Part model, mm, in its own coordinate system. A direction names the side the tool comes from. Coordinates: 2 decimals unless noted, no trailing zeros. Loops run counter-clockwise (first coordinate to the right, second up) from the corner with the lowest first, then second, coordinate; pieces in that order, holes last. Notation, with made-up numbers: (60.5, 39.25) - (77.5, 39.25) arc R30 cw to (77.5, 71.25) - close; hole circle Ø5 at (-35, -23). An arc over 180 degrees is marked (long way). Use a Markdown table: item, result. Add a question column.
1) Pull direction X, two halves, no side cores. Call faces 6 (the face through (-33.8, 24.45, -11.25)), 7 (the face through (-1, 25.25, 0)), 8 (the face through (-76.25, -5, -17)), 9 (the face through (76.25, -5, -17)): +X half, -X half, draft (parallel to the pull), parting line (faces both ways), or undercut.
2) Band-saw the part on C-C (z = -16.5). Give the cut face in (x, y), plus the area to 3 significant figures.
3) Band-saw the part on A-A (y = 1.5). Give the cut face in (x, z), plus the area to 3 significant figures.
4) Drop flat-ended pins along their axis: P1, Ø6.5, axis at x = 9, z = 0, coming from the -Y side; P2, Ø10, axis at y = 8, z = -31.5, coming from the -X side. Give the stop position or say it passes through.
5) Probe probe 1 along X at (y, z) = (-13.5, -41); probe 2 along Z at (x, y) = (-67, 1); probe 3 along Y at (x, z) = (41, 4). List the from-to ranges inside material, lowest first. Write a range as [from, to].
6) Tool access for faces 1 (the face through (-75.8, 0.8, -35.7)), 2 (the face through (75.25, 0, 0)), 3 (the face through (55, 18.07, 10.76)), 4 (the face through (-75.25, -10, -25)), 5 (the face through (-1, -21, 11.25)): list every direction of +Z, -Z, +X, -X, +Y, -Y with a clear straight run to the whole face (end or side of a thin tool).
7) Band-saw the part on D-D (y = 22.5). Give the cut face in (x, z).
8) Band-saw the part on B-B (x = 5). Give the cut face in (y, z).
from build123d import *

# Parameters (mm, degrees)
SKETCH1_W           = 150.5
SKETCH1_H           = 48.5
BOSS_EXTRUDE1_DEPTH = 10.25
SHELL1_T            = 1
SKETCH2_W           = 145.5
SKETCH2_H           = 48.5
CUT_EXTRUDE1_DEPTH  = 1
CUT_EXTRUDE2_DEPTH  = 1
BOSS_EXTRUDE2_DEPTH = 1


with BuildPart() as part:
    # Sketch1 → Boss-Extrude1 (new, symmetric)
    with BuildSketch(Plane.XY):
        Rectangle(SKETCH1_W, SKETCH1_H)
    extrude(amount=BOSS_EXTRUDE1_DEPTH, both=True)

    # Shell1
    shell1_openings = [part.faces().sort_by_distance(p)[0] for p in [
        (0, -24.25, 0),
    ]]
    offset(amount=SHELL1_T, openings=shell1_openings, kind=Kind.INTERSECTION)

    # Sketch2 → Cut-Extrude1 (cut)
    with BuildSketch(Plane(origin=(0, 0, -11.25), x_dir=(-1, 0, 0), z_dir=(0, 0, -1))):
        Rectangle(SKETCH2_W, SKETCH2_H)
    extrude(amount=-CUT_EXTRUDE1_DEPTH, mode=Mode.SUBTRACT)

    # Sketch3 → Cut-Extrude2 (cut)
    with BuildSketch(Plane.XY.offset(11.25)):
        with BuildLine():
            Line((51.5, -19.5), (-51.5, -19.5))
            ThreePointArc((-51.5, -19.5), (-55.035533906, -18.035533906), (-56.5, -14.5))
            Line((-56.5, -14.5), (-56.5, 14.5))
            ThreePointArc((-56.5, 14.5), (-55.035533906, 18.035533906), (-51.5, 19.5))
            Line((-51.5, 19.5), (51.5, 19.5))
            ThreePointArc((51.5, 19.5), (55.035533906, 18.035533906), (56.5, 14.5))
            Line((56.5, 14.5), (56.5, -14.5))
            ThreePointArc((56.5, -14.5), (55.035533906, -18.035533906), (51.5, -19.5))
        make_face()
    extrude(amount=-CUT_EXTRUDE2_DEPTH, mode=Mode.SUBTRACT)

    # Sketch4 → Boss-Extrude2 (add)
    with BuildSketch(Plane(origin=(76.25, 0, 0), x_dir=(0, 0, -1), z_dir=(1, 0, 0))):
        Polygon((11.25, 25.25), (60.75, -24.25), (11.25, -24.25), align=None)
    boss_extrude2 = extrude(amount=-BOSS_EXTRUDE2_DEPTH)

    # Mirror1: Boss-Extrude2 across plane
    add(boss_extrude2.mirror(Plane(origin=(0, 0, 0), x_dir=(0, 0, 1), z_dir=(1, 0, 0))))


solid = part.part
Answer block:
| question | item | result |
|---|---|---|
| 1 | face 6 | undercut |
| 1 | face 7 | draft |
| 1 | face 8 | -X half |
| 1 | face 9 | +X half |
| 2 | outline | (-76.25, -24.25) - (-75.25, -24.25) - (-75.25, 20) - (-76.25, 20) - close; (75.25, -24.25) - (76.25, -24.25) - (76.25, 20) - (75.25, 20) - close |
| 2 | area | 88.5 mm2 |
| 3 | outline | (-76.25, -35) - (-75.25, -35) - (-75.25, -11.25) - (-72.75, -11.25) - (-72.75, -10.25) - (-75.25, -10.25) - (-75.25, 10.25) - (-56.5, 10.25) - (-56.5, 11.25) - (-76.25, 11.25) - close; (56.5, 10.25) - (75.25, 10.25) - (75.25, -10.25) - (72.75, -10.25) - (72.75, -11.25) - (75.25, -11.25) - (75.25, -35) - (76.25, -35) - (76.25, 11.25) - (56.5, 11.25) - close |
| 3 | area | 135 mm2 |
| 4 | P1 | y = 24.25 |
| 4 | P2 | x = -76.25 |
| 5 | probe 1 | [-76.25, -75.25], [75.25, 76.25] |
| 5 | probe 2 | [10.25, 11.25] |
| 5 | probe 3 | [24.25, 25.25] |
| 6 | face 1 | -Z, +X, -X, +Y |
| 6 | face 2 | -Y |
| 6 | face 3 | +Z, -Z |
| 6 | face 4 | -Z, +Y, -Y |
| 6 | face 5 | +Z, +X, -X, +Y, -Y |
| 7 | outline | (-76.25, -14) - (-75.25, -14) - (-75.25, -11.25) - (-72.75, -11.25) - (-72.75, -10.25) - (-75.25, -10.25) - (-75.25, 10.25) - (75.25, 10.25) - (75.25, -10.25) - (72.75, -10.25) - (72.75, -11.25) - (75.25, -11.25) - (75.25, -14) - (76.25, -14) - (76.25, 11.25) - (-76.25, 11.25) - close |
| 8 | outline | (-24.25, 10.25) - (-19.5, 10.25) - (-19.5, 11.25) - (-24.25, 11.25) - close; (19.5, 10.25) - (24.25, 10.25) - (24.25, -11.25) - (25.25, -11.25) - (25.25, 11.25) - (19.5, 11.25) - close |
